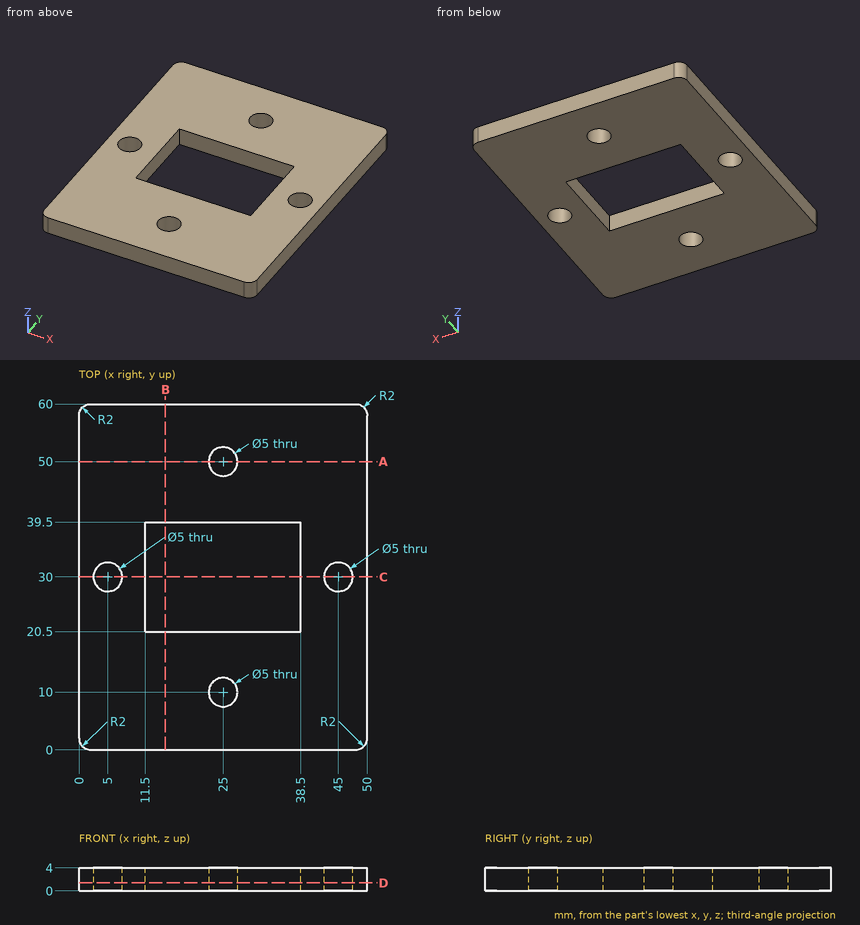
Print and shaded views of the part. All mm, measured from the part's lowest x, y and z. Give positions to 0.01 mm unless a question says otherwise; leave off trailing zeros. Loops run counter-clockwise (first coordinate to the right, second up) from the corner with the lowest first, then second, coordinate; pieces in that order, holes last. Notation, with made-up numbers: (23, -26) -> (57, -26) arc R25 cw to (57, 3) -> close; hole circle Ø8 at (80.5, -17). An arc over 180 degrees is marked (long way). Use CSV: the item, a comma, the result in double quotes. Start each with the question number.
1) Slice it at A-A on y = 50. Give the cut face in (x, z).
2) Slice it at B-B on x = 15. Give the cut face in (y, z).
3) Slice it at C-C on y = 30. Give the cut face in (x, z).
4) Wall check: line 1 (Y direction, x = 32, z = 0.6); line 2 (Y direction, x = 5, z = 1.85). Give the ranges that are in metal, low to high.
5) Slice it at D-D on z = 1.4. Give the cut face in (x, y), plus the area to 3 significant figures.
Computed values:
1,outline,"(0, 0) -> (22.5, 0) -> (22.5, 4) -> (0, 4) -> close; (27.5, 0) -> (50, 0) -> (50, 4) -> (27.5, 4) -> close"
2,outline,"(0, 0) -> (20.5, 0) -> (20.5, 4) -> (0, 4) -> close; (39.5, 0) -> (60, 0) -> (60, 4) -> (39.5, 4) -> close"
3,outline,"(0, 0) -> (2.5, 0) -> (2.5, 4) -> (0, 4) -> close; (7.5, 0) -> (11.5, 0) -> (11.5, 4) -> (7.5, 4) -> close; (38.5, 0) -> (42.5, 0) -> (42.5, 4) -> (38.5, 4) -> close; (47.5, 0) -> (50, 0) -> (50, 4) -> (47.5, 4) -> close"
4,line 1,"y = 0 to 20.5, 39.5 to 60"
4,line 2,"y = 0 to 27.5, 32.5 to 60"
5,outline,"(0, 2) arc R2 ccw to (2, 0) -> (48, 0) arc R2 ccw to (50, 2) -> (50, 58) arc R2 ccw to (48, 60) -> (2, 60) arc R2 ccw to (0, 58) -> close; hole circle Ø5 at (5, 30); hole (11.5, 20.5) -> (38.5, 20.5) -> (38.5, 39.5) -> (11.5, 39.5) -> close; hole circle Ø5 at (25, 10); hole circle Ø5 at (25, 50); hole circle Ø5 at (45, 30)"
5,area,"2,410 mm^2"
